Autodesk Inventor part; units mm, degrees
ref_plane "YZ Plane" through (0, 0, 0) normal (1, 0, 0) x (0, 1, 0)
ref_plane "XZ Plane" through (0, 0, 0) normal (0, 1, 0) x (-1, 0, 0)
ref_plane "XY Plane" through (0, 0, 0) normal (0, 0, 1) x (1, 0, 0)
sketch "スケッチ1" plane through (0, 0, 0) normal (0, 0, 1) x (1, 0, 0)
  line L0 (0, 0) -> (4, 0)
  line L1 (4, 0) -> (4, 1.5)
  line L2 (4, 1.5) -> (0, 1.5)
  line L3 (0, 1.5) -> (0, 0)
  line L4 (0, 0) -> (0, 2.75)
  line L5 (0, 0) -> (-2, 0)
  line L6 (-2, 0) -> (0, 0)
  line L7 (-2, 0) -> (-2, 1.15)
  arc A0 (0, 2.75) -> (-2, 1.15) centre (-0.0403, 0.7504) ccw
  dimension "d0" = 1.5
  dimension "d1" = 4
  dimension "d3" = 2
  dimension "d4" = 2.75
  dimension "d5" = 1.15
  dimension "d6" = 2
revolve "回転1" add sketch "スケッチ1" angle 360 about axis through (-2, 0, 0) along (1, 0, 0)
thread "ねじ1"
sketch "スケッチ2" plane through (-2, 0, 0) normal (-1, 0, 0) x (0, 0, 1)
  circle A0 centre (0, 0) radius 1.15
  line L0 (-0.575, 0.9959) -> (0.575, 0.9959)
  line L1 (0.575, 0.9959) -> (1.15, 0)
  line L2 (1.15, 0) -> (0.575, -0.9959)
  line L3 (0.575, -0.9959) -> (-0.575, -0.9959)
  line L4 (-0.575, -0.9959) -> (-1.15, 0)
  line L5 (-1.15, 0) -> (-0.575, 0.9959)
  dimension "d10" = 1.15
  dimension "d11" = 1.9919
extrude "押し出し1" cut sketch "スケッチ2" against normal blind 1.4 contours L2 L3 L4 L5 L0 L1
fillet "フィレット1" radius 0.2 6 edges at (-0.6, 0.9959, 0) (-0.6, 0.498, 0.8625) (-0.6, 0.498, -0.8625) (-0.6, -0.498, -0.8625) (-0.6, -0.9959, 0) (-0.6, -0.498, 0.8625)
fillet "フィレット2" radius 0.1 1 edges at (0, -1.5, 0)
fillet "フィレット3" radius 0.1 1 edges at (4, -1.5, 0)
properties part number "ボタンネジM3L4" material "鋼"
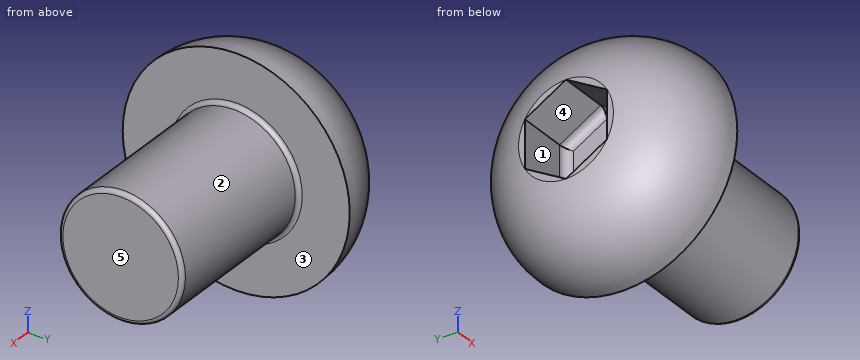
The listing builds one solid part. Answer for the finished solid, in the listing's coordinates (mm). Face numbers are marked on the shaded views. A direction names the side the tool comes from. Give positions to 0.01 mm unless a question says otherwise; leave off trailing zeros. Order: outer loops, then holes, each group sorted by start corner. A loop starts at its lowest first (then second) coordinate and runs counter-clockwise, first axis right, second up. Notation, with made-up numbers: M 82.25,37 L 104.25,37 A15 cw 104.25,58 Z; hole C 23.25,20.5 d9. An arc over 180 degrees is marked long. Put each result on its own line as item: value. Start each with the question number.
Item 1: Find the intervals of material crossed by line 1 along Y through (x, z) = (-1.6, -1.2); line 2 along Z through (x, y) = (-0.7, 0.35); line 3 along Z through (x, y) = (-1.5, -0.65), in increasing order.
Item 2: Which of the six approach directions +Z, -Z, +X, -X, +Y, -Y give full straight-line access (tool end or side, diameter ignored) to the marked faces 4 and 5?
Item 3: The part is cut by section A-A, the plane x = 3.5. Determine the outline of the cut face in (y, z), and give its area (3 significant figures).
Item 4: For a pull along Z with two mould halves and no side action, classify the marked faces 1, 2 and 3 as +Z half, -Z half, draft (parallel to the pull), parting line (faces both ways), or undercut.
Item 5: Flat-ended cylindrical pins translate along their axes: P1, Ø0.6, axis at x = -1.5, z = 0, coming from the -Y side; P2, Ø1.3, axis at x = -1.5, z = 0, coming from the +Y side; P3, Ø1.5, axis at x = 2, z = 1, coming from the +Y side; P4, Ø3, axis at y = 0, z = 1.5, coming from the +X side. Find the tip coordinate at first contact, or state that the pin passes through.
Answer key:
1. line 1: y = -1.6 to 1.6
1. line 2: z = -2.62 to -0.92, 0.92 to 2.62
1. line 3: z = -2.02 to -0.77, 0.77 to 2.02
2. face 4: -X
2. face 5: +Z, -Z, +X, +Y, -Y
3. outline: C 0,0 d3
3. area: 7.07 mm²
4. face 1: undercut
4. face 2: parting line
4. face 3: draft
5. P1: stops at y = -2.38
5. P2: stops at y = 2.58
5. P3: stops at y = 1.48
5. P4: stops at x = 4
